```python
from build123d import *

# Parameters (mm, degrees)
SKETCH_1_R          = 4.25
EXTRUDE_1_DEPTH     = 1.2
SKETCH_2_R          = 2
EXTRUDE_2_DEPTH     = 30
SKETCH_3_R          = 4.25
EXTRUDE_3_DEPTH     = 1.2
CUT_EXTRUDE_1_DEPTH = 1
CUT_EXTRUDE_2_DEPTH = 1


with BuildPart() as part:
    # 草图1 → 凸台-拉伸1 (new body)
    with BuildSketch(Plane.XY):
        Circle(SKETCH_1_R)
    extrude(amount=EXTRUDE_1_DEPTH)

    # 草图2 → 凸台-拉伸2 (add)
    with BuildSketch(Plane.XY.offset(1.2)):
        Circle(SKETCH_2_R)
    extrude(amount=EXTRUDE_2_DEPTH)

    # 草图3 → 凸台-拉伸3 (add)
    with BuildSketch(Plane.XY.offset(31.2)):
        Circle(SKETCH_3_R)
    extrude(amount=EXTRUDE_3_DEPTH)

    # 草图4 → 切除-拉伸1 (cut)
    with BuildSketch(Plane.XY.offset(32.4)):
        with BuildLine():
            Line((-0.5, 2), (-0.5, 0.5))
            Line((-0.5, 0.5), (-4.723610907, 0.5))
            ThreePointArc((-4.723610907, 0.5), (-4.75, 0), (-4.723610907, -0.5))
            Line((-4.723610907, -0.5), (-0.5, -0.5))
            Line((-0.5, -0.5), (-0.5, -2))
            Line((-0.5, -2), (0.5, -2))
            Line((0.5, -2), (0.5, -0.5))
            Line((0.5, -0.5), (4.723610907, -0.5))
            ThreePointArc((4.723610907, -0.5), (4.75, 0), (4.723610907, 0.5))
            Line((4.723610907, 0.5), (0.5, 0.5))
            Line((0.5, 0.5), (0.5, 2))
            Line((0.5, 2), (-0.5, 2))
        make_face()
    extrude(amount=-CUT_EXTRUDE_1_DEPTH, mode=Mode.SUBTRACT)

    # 草图5 → 切除-拉伸2 (cut)
    with BuildSketch(Plane(origin=(0, 0, 0), x_dir=(-1, 0, 0), z_dir=(0, 0, -1))):
        with BuildLine():
            Line((-4.723610907, -0.5), (4.723610907, -0.5))
            ThreePointArc((4.723610907, -0.5), (4.75, 0), (4.723610907, 0.5))
            Line((4.723610907, 0.5), (-4.723610907, 0.5))
            ThreePointArc((-4.723610907, 0.5), (-4.75, 0), (-4.723610907, -0.5))
        make_face()
    extrude(amount=-CUT_EXTRUDE_2_DEPTH, mode=Mode.SUBTRACT)


solid = part.part
```
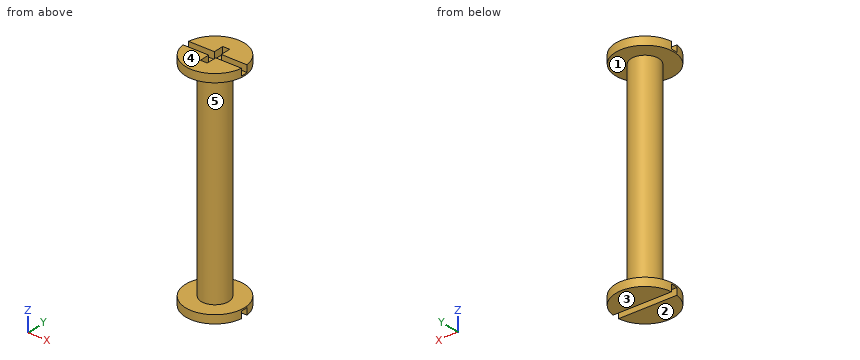
Source: CAD feature listing. Evaluate the final solid. Frame: model axes, mm. Face numbers are marked on the shaded views. A direction names the side the tool comes from. Coordinates: 2 decimals unless noted, no trailing zeros. Write each loop counter-clockwise with the first axis right and the second up, starting at its lowest first coordinate (ties: lowest second). Pieces come first, ordered by that corner, then holes. Notation, with made-up numbers: (30.25, 34) -> (65.25, 34) arc R25 cw to (65.25, 50) -> close; hole circle Ø6 at (71, -3.5). An arc over 180 degrees is marked (long way). Return JSON: item names as keys, results as strings. Group by question number.
1) Section query C-C, the plane y = -3. Return loops of the section in (x, z), plus the area to 3 significant figures.
2) Contact query for flat-ended pins moving along their axis: P1, Ø1.1, axis at y = -1, z = 32, coming from the -X side; P2, Ø5, axis at y = 2.5, z = 14.5, coming from the +X side; P3, Ø0.5, axis at x = -1.5, z = 0.5, coming from the -Y side. Output: stop coordinate, or through.
3) Section query D-D, the plane z = 6. Return loops of the section in (x, y).
4) Section query A-A, the plane x = 0. Return loops of the section in (y, z).
5) Mould query, pull axis Z, two halves, no side actions, for the marked faces 3, 4 and 5. Classes: +Z half, -Z half, draft (parallel to the pull), parting line (faces both ways), or undercut.
6) Ray query, line 1 along Z through (x, y) = (-3.5, 0.25); line 2 along Z through (x, y) = (0.25, 3.75); line 3 along Z through (x, y) = (1.75, 0.25). Return the intervals inside material, ascending.
7) Section query B-B, the plane y = 0. Return loops of the section in (x, z), plus the area to 3 significant figures.
8) Set-up query: the marked faces 1 and 2. Return all of +Z, -Z, +X, -X, +Y, -Y with unobstructed straight access to the full face (end or side cutting, diameter ignored); none if empty.
From the geometry:
{
 "1": {"outline": "(-3.01, 0) -> (3.01, 0) -> (3.01, 1.2) -> (-3.01, 1.2) -> close; (-3.01, 31.2) -> (3.01, 31.2) -> (3.01, 32.4) -> (-3.01, 32.4) -> close", "area": "14.4 mm²"},
 "2": {"P1": "x = -4.22", "P2": "x = 2", "P3": "y = -4.06"},
 "3": {"outline": "circle Ø4 at (0, 0)"},
 "4": {"outline": "(-4.25, 0) -> (-0.5, 0) -> (-0.5, 1) -> (0.5, 1) -> (0.5, 0) -> (4.25, 0) -> (4.25, 1.2) -> (2, 1.2) -> (2, 31.2) -> (4.25, 31.2) -> (4.25, 32.4) -> (2, 32.4) -> (2, 31.4) -> (-2, 31.4) -> (-2, 32.4) -> (-4.25, 32.4) -> (-4.25, 31.2) -> (-2, 31.2) -> (-2, 1.2) -> (-4.25, 1.2) -> close"},
 "5": {"face 3": "-Z half", "face 4": "+Z half", "face 5": "undercut"},
 "6": {"line 1": "1 to 1.2, 31.2 to 31.4", "line 2": "0 to 1.2, 31.2 to 32.4", "line 3": "1 to 31.4"},
 "7": {"outline": "(-4.25, 1) -> (4.25, 1) -> (4.25, 1.2) -> (2, 1.2) -> (2, 31.2) -> (4.25, 31.2) -> (4.25, 31.4) -> (-4.25, 31.4) -> (-4.25, 31.2) -> (-2, 31.2) -> (-2, 1.2) -> (-4.25, 1.2) -> close", "area": "123 mm²"},
 "8": {"face 1": "none", "face 2": "-Z, +X, -X, +Y, -Y"}
}
